from build123d import *

# Parameters (mm, degrees)
F1_W     = 22
F1_H     = 16
F2_DEPTH = 2
F3_W     = 2
F3_H     = 12
F3_W_2   = 22
F4_DEPTH = 2
F5_W     = 30
F5_H     = 16
F5_W_2   = 26
F5_H_2   = 12
F6_DEPTH = 2


with BuildPart() as f2:
    # F1 (on Top) → F2 (new body)
    with BuildSketch(Plane.XY):
        Rectangle(F1_W, F1_H)
    extrude(amount=F2_DEPTH)

    # F3 (on face) → F4 (join)
    with BuildSketch(Plane.XY.offset(2)):
        with Locations((-12, 0)):
            Rectangle(F3_W, F3_H)
        Rectangle(F3_W_2, F3_H)
        with Locations((12, 0)):
            Rectangle(F3_W, F3_H)
    extrude(amount=F4_DEPTH)

    # F5 (on face) → F6 (join)
    with BuildSketch(Plane.XY.offset(4)):
        Rectangle(F5_W, F5_H)
        Rectangle(F5_W_2, F5_H_2, mode=Mode.SUBTRACT)
        Rectangle(F5_W_2, F5_H_2)
    extrude(amount=F6_DEPTH)


solid = f2.part
Here's how the part is built. I have some questions about the finished solid (model axes, mm). A direction names the side the tool comes from. Give positions to 0.01 mm unless a question says otherwise; leave off trailing zeros. Order: outer loops, then holes, each group sorted by start corner. A loop starts at its lowest first (then second) coordinate and runs counter-clockwise, first axis right, second up. Notation, with made-up numbers: (52, 5.5) -> (78, 5.5) arc R9 cw to (78, 15.5) -> close; hole circle Ø11 at (-4.75, 69.25). An arc over 180 degrees is marked (long way). Use a Markdown table: item, result. Add a question column.
Item 1: Imagine slicing it at B-B on y = 4.25. Please give me the cut outline in (x, z), plus the area to 3 significant figures.
Item 2: For faces 4 (the face through (11, 0, 1)), 5 (the face through (-12, 0, 2)), 6 (the face through (0, -7, 4)), which set-ups out of +Z, -Z, +X, -X, +Y, -Y let a thin tool reach every point of the face, with its end or its side?
Item 3: Imagine slicing it at D-D on z = 3.3. Please give me the cut outline in (x, y).
Item 4: If we mould it in two halves opening along Z, with no side actions, what happens to faces 1 (the face through (0, -7, 2)), 2 (the face through (12, 0, 2)), 3 (the face through (0, -8, 1))? For each: pulls with the +Z half, pulls with the -Z half, needs draft (parallel to the pull), parting line crosses it, or undercut.
Item 5: Imagine slicing it at A-A on y = 6.5. Please give me the cut outline in (x, z).
Item 6: Imagine slicing it at C-C on x = -8.75. Please give me the cut outline in (y, z), plus the area to 3 significant figures.
Item 7: I need wall thicknesses on line 1 (Z direction, x = -1.5, y = 7); line 2 (X direction, y = -2.25, z = 0.3); line 3 (Y direction, x = 9.75, z = 2.35). Which ranges of each line are inside material? Lowest first, please.
Item 8: Will these pins go through, and if not, where does the flat tip stop? pin 1 (1 mm diameter, centred on x = -6, z = 3, fed in from -Y); pin 2 (1.6 mm diameter, centred on x = -5.5, z = 3, fed in from +Y); pin 3 (1.6 mm diameter, centred on x = 12, y = 2, fed in from -Z).
Data:
| question | item | result |
|---|---|---|
| 1 | outline | (-15, 4) -> (-13, 4) -> (-13, 2) -> (-11, 2) -> (-11, 0) -> (11, 0) -> (11, 2) -> (13, 2) -> (13, 4) -> (15, 4) -> (15, 6) -> (-15, 6) -> close |
| 1 | area | 156 mm² |
| 2 | face 4 | -Z, +X, +Y, -Y |
| 2 | face 5 | -Z, -X, +Y, -Y |
| 2 | face 6 | none |
| 3 | outline | (-13, -6) -> (13, -6) -> (13, 6) -> (-13, 6) -> close |
| 4 | face 1 | undercut |
| 4 | face 2 | pulls with the -Z half |
| 4 | face 3 | needs draft |
| 5 | outline | (-15, 4) -> (15, 4) -> (15, 6) -> (-15, 6) -> close; (-11, 0) -> (11, 0) -> (11, 2) -> (-11, 2) -> close |
| 6 | outline | (-8, 0) -> (8, 0) -> (8, 2) -> (6, 2) -> (6, 4) -> (8, 4) -> (8, 6) -> (-8, 6) -> (-8, 4) -> (-6, 4) -> (-6, 2) -> (-8, 2) -> close |
| 6 | area | 88.0 mm² |
| 7 | line 1 | z = 0 to 2, 4 to 6 |
| 7 | line 2 | x = -11 to 11 |
| 7 | line 3 | y = -6 to 6 |
| 8 | pin 1 | stops at y = -6 |
| 8 | pin 2 | stops at y = 6 |
| 8 | pin 3 | stops at z = 2 |
